from build123d import *

# Parameters (mm, degrees)
F1_DEPTH = 2438.4
F3_DEPTH = 1229.2


with BuildPart() as f1:
    # F0 (on Right) → F1 (new body)
    with BuildSketch(Plane.YZ):
        Polygon((0, 50.8), (0, 0), (50.8, 0), (50.8, 5), (5, 5), (5, 50.8), align=None)
        Polygon((1229.2, 0), (1229.2, 50.8), (1224.2, 50.8), (1224.2, 5), (1178.4, 5), (1178.4, 0), align=None)
    extrude(amount=F1_DEPTH)

    # F2 (on Front) → F3 (join, through all)
    with BuildSketch(Plane.XZ):
        Polygon((152.4, 0), (101.6, 0), (101.6, -50.8), (106.6, -50.8), (106.6, -5), (152.4, -5), align=None)
        Polygon((868.6, -50.8), (868.6, -5), (914.4, -5), (914.4, 0), (863.6, 0), (863.6, -50.8), align=None)
        Polygon((1630.6, -50.8), (1630.6, -5), (1676.4, -5), (1676.4, 0), (1625.6, 0), (1625.6, -50.8), align=None)
        Polygon((2392.6, -50.8), (2392.6, -5), (2438.4, -5), (2438.4, 0), (2387.6, 0), (2387.6, -50.8), align=None)
    extrude(amount=-F3_DEPTH)


solid = f1.part
Geometry check sheet. Reference: the model listing, model coordinates, mm. A direction names the side the tool comes from. Round coordinates to 2 decimals unless told otherwise and drop trailing zeros. Write each loop counter-clockwise with the first axis right and the second up, starting at its lowest first coordinate (ties: lowest second). Pieces come first, ordered by that corner, then holes. Notation, with made-up numbers: (-19.5, -13) - (5.5, -13) arc R24 ccw to (5.5, 25) - close; hole circle Ø2 at (-39, -10). An arc over 180 degrees is marked (long way). One line per item, written item: value.
1. Set-up check for faces 1 (the face through (1202, 1202, 5)), 2 (the face through (106.6, 606, -28)), 3 (the face through (50, 1203, 0)): record each of +Z, -Z, +X, -X, +Y, -Y from which the full face is reachable in a straight line by a thin tool's end or side.
The answers:
face 1: +Z, +X, -X
face 2: -Z, +Y, -Y
face 3: -Z, -X, +Y, -Y
2. Mould release check, pull along X, two halves, no side actions. Record for faces 4 (the face through (1265, 1203, 0)), 5 (the face through (1202, 1229.2, 23)), 6 (the face through (0, 1215, 4.8)): released by +X, released by -X, zero draft, split by the parting line, or undercut.
The answers:
face 4: undercut
face 5: zero draft
face 6: released by -X
3. Cross-section at A-A on x = 326.5. Record the boundary of the cut face in (y, z), and give its area (3 significant figures).
The answers:
outline: (0, 0) - (50.8, 0) - (50.8, 5) - (5, 5) - (5, 50.8) - (0, 50.8) - close; (1178.4, 0) - (1229.2, 0) - (1229.2, 50.8) - (1224.2, 50.8) - (1224.2, 5) - (1178.4, 5) - close
area: 966 mm^2
4. Depth check by flat-ended pin: pin 1 Ø5 at (y, z) = (425.5, -9.5) entering from -X; pin 2 Ø15 at (x, y) = (663.5, 1209.5) entering from -Z; pin 3 Ø13.5 at (y, z) = (568.5, -17.5) entering from +X. Enter the tip coordinate at first touch or a pass-through.
The answers:
pin 1: stops at x = 101.6
pin 2: stops at z = 0
pin 3: stops at x = 2392.6
5. Scan lines: L1, parallel to X at y = 349, z = -18; L2, parallel to X at y = 176, z = -2.5; L3, parallel to Y at x = 831, z = 0.5. Record each from-to range of solid material in increasing order.
The answers:
L1: x = 101.6 to 106.6, 863.6 to 868.6, 1625.6 to 1630.6, 2387.6 to 2392.6
L2: x = 101.6 to 152.4, 863.6 to 914.4, 1625.6 to 1676.4, 2387.6 to 2438.4
L3: y = 0 to 50.8, 1178.4 to 1229.2
6. Cross-section at B-B on z = -22.5. Record the boundary of the cut face in (x, y).
The answers:
outline: (101.6, 0) - (106.6, 0) - (106.6, 1229.2) - (101.6, 1229.2) - close; (863.6, 0) - (868.6, 0) - (868.6, 1229.2) - (863.6, 1229.2) - close; (1625.6, 0) - (1630.6, 0) - (1630.6, 1229.2) - (1625.6, 1229.2) - close; (2387.6, 0) - (2392.6, 0) - (2392.6, 1229.2) - (2387.6, 1229.2) - close
7. Cross-section at C-C on y = 194. Record the boundary of the cut face in (x, z), and give its area (3 significant figures).
The answers:
outline: (101.6, -50.8) - (106.6, -50.8) - (106.6, -5) - (152.4, -5) - (152.4, 0) - (101.6, 0) - close; (863.6, -50.8) - (868.6, -50.8) - (868.6, -5) - (914.4, -5) - (914.4, 0) - (863.6, 0) - close; (1625.6, -50.8) - (1630.6, -50.8) - (1630.6, -5) - (1676.4, -5) - (1676.4, 0) - (1625.6, 0) - close; (2387.6, -50.8) - (2392.6, -50.8) - (2392.6, -5) - (2438.4, -5) - (2438.4, 0) - (2387.6, 0) - close
area: 1,930 mm^2
